```python
from build123d import *

# Parameters (mm, degrees)
SKETCH_1_W          = 50
SKETCH_1_H          = 40
EXTRUDE_1_DEPTH     = 15
SKETCH_2_R          = 1.6
CUT_EXTRUDE_1_DEPTH = 36.355339059
FILLET_1_R          = 15
FILLET_2_R          = 1
FILLET_3_R          = 1


with BuildPart() as part:
    # 草图1 → 凸台-拉伸1 (new body)
    with BuildSketch(Plane.XY):
        Rectangle(SKETCH_1_W, SKETCH_1_H)
    extrude(amount=EXTRUDE_1_DEPTH)

    # 草图2 → 切除-拉伸1 (cut, through all)
    with BuildSketch(Plane.XY.offset(15)):
        with Locations((-10, 10)):
            Circle(SKETCH_2_R)
        with Locations(Location((15, 10, 0), (0, 0, 180))):
            Circle(SKETCH_2_R)
        with Locations((15, -10)):
            Circle(SKETCH_2_R)
        with Locations(Location((-10, -10, 0), (0, 0, 180))):
            Circle(SKETCH_2_R)
    extrude(amount=-CUT_EXTRUDE_1_DEPTH, mode=Mode.SUBTRACT)

    # 圆角1
    fillet_1_edges = [part.edges().sort_by_distance(p)[0] for p in [
        (25, -20, 7.5),
        (25, 20, 7.5),
    ]]
    fillet(fillet_1_edges, radius=FILLET_1_R)

    # 圆角2
    fillet_2_edges = [part.edges().sort_by_distance(p)[0] for p in [
        (-25, -20, 7.5),
        (-25, 20, 7.5),
    ]]
    fillet(fillet_2_edges, radius=FILLET_2_R)

    # 圆角3
    fillet_3_edges = [part.edges().sort_by_distance(p)[0] for p in [
        (25, 0, 0),
        (25, 0, 15),
        (-7, 20, 0),
        (20.606601718, 15.606601718, 0),
        (20.606601718, -15.606601718, 0),
        (-7, 20, 15),
        (20.606601718, 15.606601718, 15),
        (20.606601718, -15.606601718, 15),
        (-7, -20, 0),
        (-7, -20, 15),
        (-25, 0, 0),
        (-24.707106781, 19.707106781, 0),
        (-24.707106781, -19.707106781, 0),
        (-25, 0, 15),
        (-24.707106781, 19.707106781, 15),
        (-24.707106781, -19.707106781, 15),
    ]]
    fillet(fillet_3_edges, radius=FILLET_3_R)


solid = part.part
```
CAD build for the part. Positions are in the model's coordinates, mm. Coordinates: 2 decimals unless noted, no trailing zeros. Loops run counter-clockwise (first coordinate to the right, second up) from the corner with the lowest first, then second, coordinate; pieces in that order, holes last. Notation, with made-up numbers: (33.5, -6) - (47.5, -6) arc R30 cw to (47.5, 20) - close; hole circle Ø2 at (74, 57). An arc over 180 degrees is marked (long way). Return JSON: item names as keys, results as strings.
1. Band-saw the part on B-B (z = 8.5). Give the cut face in (x, y), and give its area (3 significant figures).
Result:
{"outline": "(-25, -19) arc R1 ccw to (-24, -20) - (10, -20) arc R15 ccw to (25, -5) - (25, 5) arc R15 ccw to (10, 20) - (-24, 20) arc R1 ccw to (-25, 19) - close; hole circle Ø3.2 at (-10, -10); hole circle Ø3.2 at (-10, 10); hole circle Ø3.2 at (15, -10); hole circle Ø3.2 at (15, 10)", "area": "1,870 mm2"}
2. Mould opens along X. For faces 1 (the cylindrical face through (-6.762, -19.699, 0.285)), 2 (the cylindrical face through (24.699, 0.07, 14.715)), 3 (the cylindrical face through (-8.4, -10.07, 7.6)) say: released by +X, released by -X, zero draft, split by the parting line, or undercut.
Result:
{"face 1": "zero draft", "face 2": "released by +X", "face 3": "undercut"}
3. Probe L1, parallel to Y at x = -10, z = 4.75; L2, parallel to X at y = -9, z = 6; L3, parallel to Y at x = 15, z = 4. List the from-to ranges inside material, lowest first. Write a range as from..to.
Result:
{"L1": "y = -20..-11.6, -8.4..8.4, 11.6..20", "L2": "x = -25..-11.25, -8.75..13.75, 16.25..24.46", "L3": "y = -19.14..-11.6, -8.4..8.4, 11.6..19.14"}
4. Drop flat-ended pins along their axis: pin 1 (1 mm diameter, centred on y = 11.5, z = 3, fed in from +X); pin 2 (1.9 mm diameter, centred on x = 15, y = -10, fed in from +Z). Give the stop position or say it passes through.
Result:
{"pin 1": "stops at x = 23.75", "pin 2": "passes through"}
5. Band-saw the part on A-A (x = -10). Give the cut face in (y, z).
Result:
{"outline": "(-20, 1) arc R1 ccw to (-19, 0) - (-11.6, 0) - (-11.6, 15) - (-19, 15) arc R1 ccw to (-20, 14) - close; (-8.4, 0) - (8.4, 0) - (8.4, 15) - (-8.4, 15) - close; (11.6, 0) - (19, 0) arc R1 ccw to (20, 1) - (20, 14) arc R1 ccw to (19, 15) - (11.6, 15) - close"}
